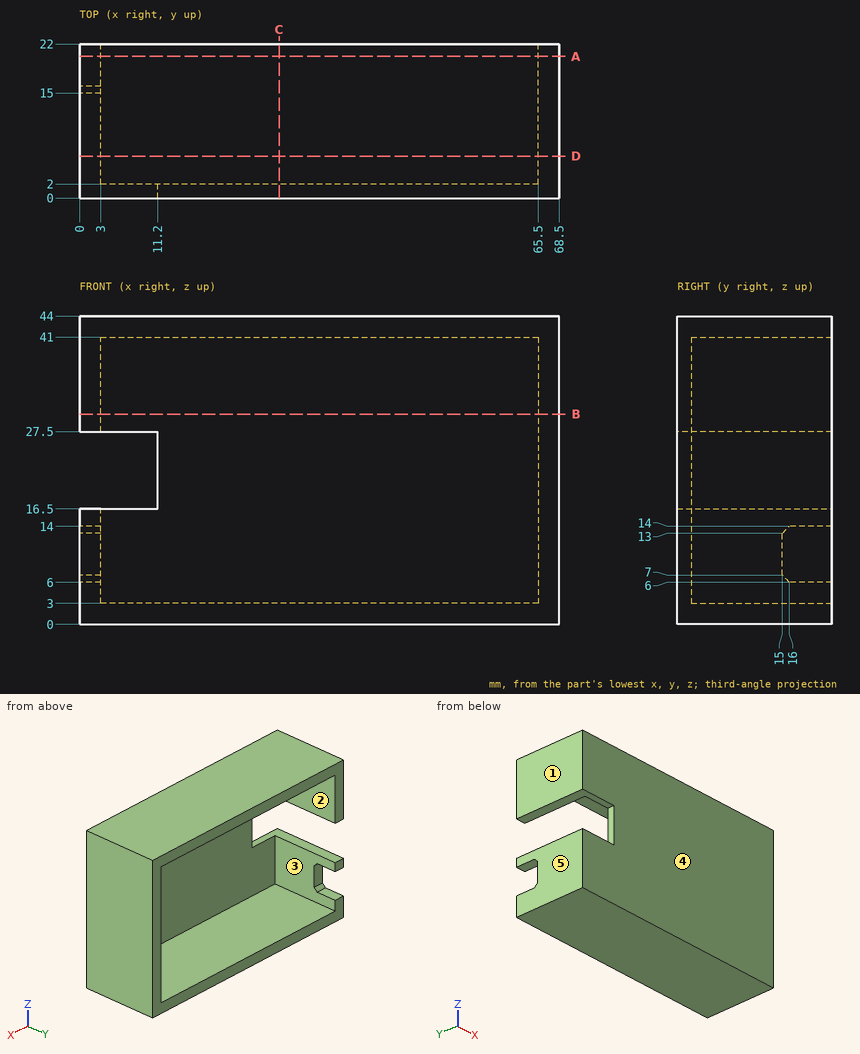
Geometry: see drawing. Coordinates: mm, zero at the bounding-box minimum. A direction names the side the tool comes from. Give positions to 0.01 mm unless a question says otherwise; leave off trailing zeros. Loops run counter-clockwise (first coordinate to the right, second up) from the corner with the lowest first, then second, coordinate; pieces in that order, holes last. Notation, with made-up numbers: (-39, -4.5) - (-4, -4.5) arc R12 ccw to (-4, 12.5) - close; hole circle Ø10 at (4, 8.25). An arc over 180 degrees is marked (long way). Answer as CSV lines item,"result". Start each with the question number.
1. Section B-B, the plane z = 30. Return loops of the section in (x, y), plus the area to 3 significant figures.
2. Section C-C, the plane x = 28.5. Return loops of the section in (y, z).
3. Section D-D, the plane y = 6. Return loops of the section in (x, z).
4. Reachability of the marked faces 1 and 2 from +Z, -Z, +X, -X, +Y, -Y: full face, straight path, thin tool, end or side. Return the list, or none.
5. Section A-A, the plane y = 20.25. Return loops of the section in (x, z), plus the area to 3 significant figures.
6. Ray query, L1, parallel to Z at x = 64.5, y = 15.5; L2, parallel to X at y = 20.75, z = 40; L3, parallel to Y at x = 26, z = 20. Return the intervals inside material, ascending.
7. Draft query along X for the marked faces 3, 4 and 5. Return one class per face: released by +X, released by -X, zero draft, split by the parting line, or undercut.
8. Pin query (flat end, axial travel): P1, Ø3.5, axis at x = 1, y = 19.5, coming from the -Z side; P2, Ø1, axis at y = 1, z = 22, coming from the -X side; P3, Ø0.9, axis at x = 2, z = 10.5, coming from the +Y side; P4, Ø3, axis at x = 30, z = 24, coming from the +Y side. Return the tip coordinate at first contact, or that it passes through.
Answers:
1,outline,"(0, 0) - (68.5, 0) - (68.5, 22) - (65.5, 22) - (65.5, 2) - (3, 2) - (3, 22) - (0, 22) - close"
1,area,"257 mm2"
2,outline,"(0, 0) - (22, 0) - (22, 3) - (2, 3) - (2, 41) - (22, 41) - (22, 44) - (0, 44) - close"
3,outline,"(0, 0) - (68.5, 0) - (68.5, 44) - (0, 44) - (0, 27.5) - (3, 27.5) - (3, 41) - (65.5, 41) - (65.5, 3) - (3, 3) - (3, 16.5) - (0, 16.5) - close"
4,face 1,"+Z, -Z, -X, +Y, -Y"
4,face 2,"+Y"
5,outline,"(0, 0) - (68.5, 0) - (68.5, 44) - (0, 44) - (0, 27.5) - (3, 27.5) - (3, 41) - (65.5, 41) - (65.5, 3) - (3, 3) - (3, 6) - (0, 6) - close; (0, 14) - (3, 14) - (3, 16.5) - (0, 16.5) - close"
5,area,"582 mm2"
6,L1,"z = 0 to 3, 41 to 44"
6,L2,"x = 0 to 3, 65.5 to 68.5"
6,L3,"y = 0 to 2"
7,face 3,"undercut"
7,face 4,"zero draft"
7,face 5,"released by -X"
8,P1,"stops at z = 0"
8,P2,"stops at x = 11.2"
8,P3,"stops at y = 15"
8,P4,"stops at y = 2"
